Verification items for the finished model (mm, model axes). Coordinates: 2 decimals unless noted, no trailing zeros. Write each loop counter-clockwise with the first axis right and the second up, starting at its lowest first coordinate (ties: lowest second). Pieces come first, ordered by that corner, then holes. Notation, with made-up numbers: M 64,-40 L 99,-40 A13 ccw 99,-19 Z; hole C 13.25,30 d8. An arc over 180 degrees is marked long. One line per item, written item: value.
```python
from build123d import *

# Parameters (mm, degrees)
SKETCH1_R           = 16.6
BOSS_EXTRUDE1_DEPTH = 16.3
CUT_EXTRUDE1_DEPTH  = 29.579888033
SKETCH3_R           = 7.7
CUT_EXTRUDE2_DEPTH  = 29.579888033
SKETCH4_W           = 0.6
SKETCH4_H           = 9.511954595
SKETCH4_W_2         = 10.341543893
SKETCH4_H_2         = 0.6
CUT_EXTRUDE3_DEPTH  = 29.579888207


with BuildPart() as part:
    # Sketch1 → Boss-Extrude1 (new body)
    with BuildSketch(Plane.XY):
        Circle(SKETCH1_R)
    extrude(amount=BOSS_EXTRUDE1_DEPTH)

    # Sketch2 → Cut-Extrude1 (cut, through all)
    with BuildSketch(Plane.XY.offset(16.3)):
        with BuildLine():
            Line((0, 0), (16.6, 0))
            ThreePointArc((16.6, 0), (-11.737972568, 11.737972568), (0, -16.6))
            Line((0, -16.6), (0, 0))
        make_face()
    extrude(amount=-CUT_EXTRUDE1_DEPTH, mode=Mode.SUBTRACT)

    # Sketch3 → Cut-Extrude2 (cut, through all)
    with BuildSketch(Plane(origin=(0, 0, 0), x_dir=(1, 0, 0), z_dir=(0, 1, 0))):
        Circle(SKETCH3_R)
    extrude(amount=-CUT_EXTRUDE2_DEPTH, mode=Mode.SUBTRACT)

    # Sketch4 → Cut-Extrude3 (cut, through all)
    with BuildSketch(Plane(origin=(0, 0, 0), x_dir=(1, 0, 0), z_dir=(0, 1, 0))):
        with Locations((0.3, -11.544022703)):
            Rectangle(SKETCH4_W, SKETCH4_H)
        with Locations((11.429228054, -0.3)):
            Rectangle(SKETCH4_W_2, SKETCH4_H_2)
    extrude(amount=-CUT_EXTRUDE3_DEPTH, mode=Mode.SUBTRACT)


solid = part.part
```
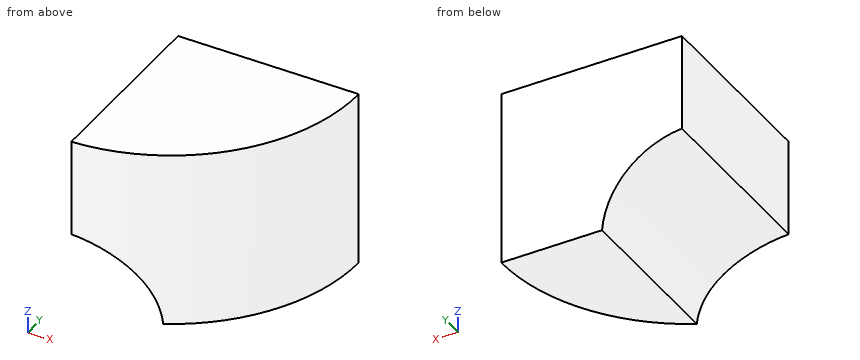
Item 1: Cross-section at D-D, the plane y = -4. Enter the section's corners in (x, z).
The answers:
outline: M 0.6,7.68 A7.7 cw 7.68,0.6 L 16.11,0.6 L 16.11,16.3 L 0.6,16.3 Z
Item 2: Cross-section at A-A, the plane y = -8.25. Enter the section's corners in (x, z), and give its area (3 significant figures).
The answers:
outline: M 0.6,7.68 A7.7 cw 7.68,0.6 L 14.4,0.6 L 14.4,16.3 L 0.6,16.3 Z
area: 179 mm²
Item 3: Cross-section at C-C, the plane z = 6.5. Enter the section's corners in (x, y).
The answers:
outline: M 4.13,-16.08 A16.6 ccw 16.6,0 L 4.13,0 Z
Item 4: Go/stop test with a flat-tipped pin: P1, Ø5, axis at y = -12, z = 10, coming from the +X side. Record where the tip stops, or that it passes through.
The answers:
P1: stops at x = 13.61
Item 5: Scan lines: line 1 (X direction, y = -1, z = 11); line 2 (Y direction, x = 11.5, z = 8); line 3 (X direction, y = -12.75, z = 11.5). Record each from-to range of solid material in increasing order.
The answers:
line 1: x = 0.6 to 16.57
line 2: y = -11.97 to 0
line 3: x = 0.6 to 10.63
Item 6: Cross-section at B-B, the plane x = 14.25. Enter the section's corners in (y, z), and give its area (3 significant figures).
The answers:
outline: M -8.51,0.6 L 0,0.6 L 0,16.3 L -8.51,16.3 Z
area: 134 mm²
